Build history of the part. All positions in model axes, mm. Round coordinates to 2 decimals unless told otherwise and drop trailing zeros. Write each loop counter-clockwise with the first axis right and the second up, starting at its lowest first coordinate (ties: lowest second). Pieces come first, ordered by that corner, then holes. Notation, with made-up numbers: (73, 40.25) - (122, 40.25) arc R14 cw to (122, 47.25) - close; hole circle Ø2 at (25, 60). An arc over 180 degrees is marked (long way). Write each question's results on one line, items separated by ' | '.
from build123d import *

# Parameters (mm, degrees)
SKETCH_1_W          = 180
SKETCH_1_H          = 180
EXTRUDE_1_DEPTH     = 2
CUT_EXTRUDE_1_DEPTH = 140
SKETCH_3_R          = 2.2
CUT_EXTRUDE_2_DEPTH = 160


with BuildPart() as part:
    # ｽｹｯﾁ1 → ﾎﾞｽ - 押し出し1 (new body)
    with BuildSketch(Plane.XY):
        Rectangle(SKETCH_1_W, SKETCH_1_H)
    extrude(amount=EXTRUDE_1_DEPTH)

    # ｽｹｯﾁ2 → ｶｯﾄ - 押し出し1 (cut)
    with BuildSketch(Plane.XY.offset(2)):
        with BuildLine():
            ThreePointArc((-52.2, -82.5), (-51.555634919, -84.055634919), (-50, -84.7))
            Line((-50, -84.7), (-50, -82.5))
            Line((-50, -82.5), (-52.2, -82.5))
        make_face()
        with BuildLine():
            Line((-50, -82.5), (-50, -84.7))
            ThreePointArc((-50, -84.7), (-48.444365081, -84.055634919), (-47.8, -82.5))
            ThreePointArc((-47.8, -82.5), (-50, -80.3), (-52.2, -82.5))
            Line((-52.2, -82.5), (-50, -82.5))
        make_face()
        with BuildLine():
            ThreePointArc((52.2, -82.5), (48.444365081, -80.944365081), (50, -84.7))
            Line((50, -84.7), (50, -82.5))
            Line((50, -82.5), (52.2, -82.5))
        make_face()
        with BuildLine():
            Line((50, -82.5), (50, -84.7))
            ThreePointArc((50, -84.7), (51.555634919, -84.055634919), (52.2, -82.5))
            Line((52.2, -82.5), (50, -82.5))
        make_face()
    extrude(amount=-CUT_EXTRUDE_1_DEPTH, mode=Mode.SUBTRACT)

    # ｽｹｯﾁ3 → ｶｯﾄ - 押し出し2 (cut)
    with BuildSketch(Plane.XY.offset(2)):
        with Locations((-82.5, 50)):
            Circle(SKETCH_3_R)
        with Locations((82.5, 50)):
            Circle(SKETCH_3_R)
        with Locations((82.5, -70)):
            Circle(SKETCH_3_R)
        with Locations((-82.5, -70)):
            Circle(SKETCH_3_R)
    extrude(amount=-CUT_EXTRUDE_2_DEPTH, mode=Mode.SUBTRACT)


solid = part.part
(1) Flat gauge pin, fed straight in: pin 1 Ø12 at (x, y) = (14, -62) entering from -Z. Where does the tip first touch, or does it go through?
Worked answers:
pin 1: stops at z = 0
(2) Two-plate mould, pull along Y, no slides. Class faces 1 (the cylindrical face through (-80.4, -69.34, 1.01)), 2 (the flat face through (-1, 1, 0)): released by +Y, released by -Y, zero draft, split by the parting line, or undercut.
Worked answers:
face 1: undercut | face 2: zero draft
(3) Slice it at A-A, the plane x = 82.5. Write the cut outline in (y, z), and give its area (3 significant figures).
Worked answers:
outline: (-90, 0) - (-72.2, 0) - (-72.2, 2) - (-90, 2) - close; (-67.8, 0) - (47.8, 0) - (47.8, 2) - (-67.8, 2) - close; (52.2, 0) - (90, 0) - (90, 2) - (52.2, 2) - close | area: 342 mm2
(4) Slice it at B-B, the plane y = 50. Write the cut outline in (x, z).
Worked answers:
outline: (-90, 0) - (-84.7, 0) - (-84.7, 2) - (-90, 2) - close; (-80.3, 0) - (80.3, 0) - (80.3, 2) - (-80.3, 2) - close; (84.7, 0) - (90, 0) - (90, 2) - (84.7, 2) - close
(5) Drill centre lines: probe 1 along Y at (x, z) = (-82.5, 1.45); probe 2 along X at (y, z) = (-82.5, 1.1); probe 3 along Y at (x, z) = (-81.5, 0.3). Where is each one in solid material? Low to high. Write a range as [from, to].
Worked answers:
probe 1: y = [-90, -72.2], [-67.8, 47.8], [52.2, 90] | probe 2: x = [-90, -52.2], [-47.8, 47.8], [52.2, 90] | probe 3: y = [-90, -71.96], [-68.04, 48.04], [51.96, 90]
